Part model, mm, in its own coordinate system. Coordinates: 2 decimals unless noted, no trailing zeros. Loops run counter-clockwise (first coordinate to the right, second up) from the corner with the lowest first, then second, coordinate; pieces in that order, holes last. Notation, with made-up numbers: (39, 71) - (89, 71) arc R18 ccw to (89, 80) - close; hole circle Ø9 at (3, 85). An arc over 180 degrees is marked (long way). Use a Markdown table: item, result. Add a question column.
1) Probe probe 1 along Y at (x, z) = (21, 0.6); probe 2 along Y at (x, z) = (32.5, 2.45); probe 3 along Y at (x, z) = (-3.5, 1.25). List the from-to ranges inside material, lowest first. Write a range as [from, to].
2) Band-saw the part on A-A (x = -6.5). Give the cut face in (y, z) (3 decimals), plus the area to 3 significant figures.
3) Drop flat-ended pins along their axis: P1, Ø1, axis at y = 4, z = 0.5, coming from the +X side; P2, Ø1.6, axis at x = 26, z = 2, coming from the -Y side; P3, Ø6, axis at x = 40.46, y = 60.91, coming from the +Z side. Give the stop position or say it passes through.
4) Band-saw the part on D-D (x = 0). Give the cut face in (y, z) (1 decimal).
5) Band-saw the part on C-C (x = 41). Give the cut face in (y, z) (3 decimals).
6) Band-saw the part on B-B (y = 0). Give the cut face in (x, z) (1 decimal).
from build123d import *

# Parameters (mm, degrees)
SKETCH1_R           = 7.9375
SKETCH1_R_2         = 3.3655
SKETCH1_R_3         = 4.191
BOSS_EXTRUDE1_DEPTH = 3.175
CUT_EXTRUDE1_DEPTH  = 6.35
FILLET1_R           = 3.175
FILLET5_R           = 7.62


with BuildPart() as part:
    # Sketch1 → Boss-Extrude1 (new body)
    with BuildSketch(Plane.XY):
        with BuildLine():
            Line((8.990505701, 142.507164257), (49.453246099, 65.638340515))
            ThreePointArc((49.453246099, 65.638340515), (50.622740399, 60.905856258), (49.453246099, 56.173372001))
            Line((49.453246099, 56.173372001), (8.177790267, -11.326281223))
            ThreePointArc((8.177790267, -11.326281223), (-6.360706327, -12.437938536), (-13.97, 0))
            ThreePointArc((-13.97, 0), (7.91990549, 68.33468047), (-10.16, 137.77468))
            ThreePointArc((-10.16, 137.77468), (-2.437423033, 147.637974022), (8.990505701, 142.507164257))
        make_face()
        Circle(SKETCH1_R, mode=Mode.SUBTRACT)
        with Locations((40.462740399, 60.905856258)):
            Circle(SKETCH1_R_2, mode=Mode.SUBTRACT)
        with Locations((0, 137.77468)):
            Circle(SKETCH1_R_3, mode=Mode.SUBTRACT)
    extrude(amount=BOSS_EXTRUDE1_DEPTH)

    # Sketch2 → Cut-Extrude1 (cut)
    with BuildSketch(Plane.XY.offset(3.175)):
        with BuildLine():
            ThreePointArc((-0.124257687, 11.111805266), (6.119551738, 9.275707131), (10.264347662, 4.258030452))
            Line((10.264347662, 4.258030452), (31.313727824, 38.681050934))
            Line((31.313727824, 38.681050934), (1.961287607, 15.442397513))
            ThreePointArc((1.961287607, 15.442397513), (0.937773258, 13.267826895), (-0.124257687, 11.111805266))
        make_face()
        with BuildLine():
            Line((6.763206822, 27.343322009), (40.914079215, 54.38094756))
            ThreePointArc((40.914079215, 54.38094756), (40.688544415, 54.369255246), (40.462740399, 54.365356258))
            Line((40.462740399, 54.365356258), (13.177274796, 54.365356258))
            ThreePointArc((13.177274796, 54.365356258), (10.666365072, 40.689104041), (6.763206822, 27.343322009))
        make_face()
        with BuildLine():
            Line((14.227692925, 66.924652484), (40.332379532, 67.445056996))
            Line((40.332379532, 67.445056996), (12.691282428, 92.804736539))
            ThreePointArc((12.691282428, 92.804736539), (14.081637817, 79.901629399), (14.227692925, 66.924652484))
        make_face()
        with BuildLine():
            Line((10.611239694, 103.330724773), (36.257061309, 79.801636355))
            Line((36.257061309, 79.801636355), (6.979807085, 135.420906636))
            ThreePointArc((6.979807085, 135.420906636), (4.67858985, 132.085325641), (0.961351613, 130.471683418))
            ThreePointArc((0.961351613, 130.471683418), (6.511625183, 117.159092878), (10.611239694, 103.330724773))
        make_face()
    extrude(amount=-CUT_EXTRUDE1_DEPTH, mode=Mode.SUBTRACT)

    # Fillet1
    # the kernel refuses this fillet: 3.175 mm, written as the material it adds along each edge
    with BuildSketch(Plane(origin=(1.961287607, 15.442397513, 3.175), x_dir=(-0.42030668038784, -0.9073821104812206, 0), z_dir=(0, 0, -1))) as fillet1_piece_1:
        with BuildLine():
            CenterArc((0.755742265, -3.174987871), FILLET1_R, 90.158373023, 26.618624782)
            Line((-0.674656078, -0.340453415), (0, 0))
            ThreePointArc((0, 0), (0.373483081, -0.000516178), (0.746966162, 0))
        make_face()
    extrude(amount=3.175)
    with BuildSketch(Plane(origin=(-0.124257687, 11.111805266, 3.175), x_dir=(0.4359761911813302, 0.8999581994309626, 0), z_dir=(0, 0, -1))) as fillet1_piece_2:
        with BuildLine():
            CenterArc((4.22998716, 3.174619998), FILLET1_R, 172.83641486, 96.277116616)
            ThreePointArc((1.07977071, 3.570550945), (0.690776023, 1.739644609), (0, 0))
            ThreePointArc((0, 0), (2.090433086, 0.016171698), (4.180866173, 0))
        make_face()
    extrude(amount=3.175)
    with BuildSketch(Plane(origin=(10.264347662, 4.258030452, 3.175), x_dir=(0.5216861951219568, 0.853137453063207, 0), z_dir=(0, 0, -1))) as fillet1_piece_3:
        with BuildLine():
            CenterArc((4.899209013, -3.175), FILLET1_R, 90, 103.603922827)
            ThreePointArc((1.813283958, -3.921787493), (1.099083544, -1.871916155), (0, 0))
            Line((0, 0), (4.899209013, 0))
        make_face()
    extrude(amount=3.175)
    with BuildSketch(Plane(origin=(31.313727824, 38.681050934, 3.175), x_dir=(-0.7840288614357019, -0.6207243707442435, 0), z_dir=(0, 0, -1))) as fillet1_piece_4:
        with BuildLine():
            CenterArc((FILLET1_R * 5.61807899766, -FILLET1_R), FILLET1_R, 90, 159.814477423)
            Line((FILLET1_R * 5.27301794688, -FILLET1_R * 1.9385802423), (0, 0))
            Line((0, 0), (FILLET1_R * 5.61807899766, 0))
        make_face()
    extrude(amount=3.175)
    with BuildSketch(Plane(origin=(40.914079215, 54.38094756, 3.175), x_dir=(-0.9999985466583668, -0.0017048991624346568, 0), z_dir=(0, 0, -1))) as fillet1_piece_5:
        with BuildLine():
            CenterArc((9.150412322, -3.174995386), FILLET1_R, 90.097683574, 141.630948821)
            Line((7.1838593, -5.667643418), (6.987203998, -5.916908221))
            Line((6.987203998, -5.916908221), (-0.196655302, -0.249264803))
            Line((-0.196655302, -0.249264803), (0.021369604, 0.316780034))
            ThreePointArc((0.021369604, 0.316780034), (0.450823437, 0.302677747), (9.144457961, 0.317499539))
            Line((9.144457961, 0.317499539), (9.144999267, 0))
        make_face()
    extrude(amount=3.175)
    with BuildSketch(Plane(origin=(6.763206822, 27.343322009, 3.175), x_dir=(0.29421486221715376, 0.9557393027654252, 0), z_dir=(0, 0, -1))) as fillet1_piece_6:
        with BuildLine():
            CenterArc((10.215496918, 3.172783065), FILLET1_R, 124.520485767, 143.338263429)
            Line((8.41622168, 5.788740561), (0, 0))
            ThreePointArc((0, 0), (5.048434414, 0.094345715), (10.096868828, 0))
        make_face()
    extrude(amount=3.175)
    with BuildSketch(Plane(origin=(13.177274796, 54.365356258, 3.175), x_dir=(-0.1397274976091422, -0.9901899951079526, 0), z_dir=(0, 0, -1))) as fillet1_piece_7:
        with BuildLine():
            CenterArc((2.758448164, -3.174838407), FILLET1_R, 90.57806828, 81.3898537)
            Line((-0.38540507, -2.731203602), (0, 0))
            ThreePointArc((0, 0), (1.363207757, -0.006876893), (2.726415514, 0))
        make_face()
    extrude(amount=3.175)
    with BuildSketch(Plane(origin=(12.691282428, 92.804736539, 3.175), x_dir=(0.12348134501551586, -0.992346893698549, 0), z_dir=(0, 0, -1))) as fillet1_piece_8:
        with BuildLine():
            CenterArc((8.634113181, -3.173416471), FILLET1_R, 91.809659599, 137.818629886)
            Line((6.577526563, -5.59231632), (0, 0))
            ThreePointArc((0, 0), (4.266924504, -0.06738998), (8.533849008, 0))
        make_face()
    extrude(amount=3.175)
    with BuildSketch(Plane(origin=(14.227692925, 66.924652484, 3.175), x_dir=(0.024643115282951916, 0.9996963123214726, 0), z_dir=(0, 0, -1))) as fillet1_piece_9:
        with BuildLine():
            CenterArc((3.319776694, 3.174765946), FILLET1_R, 177.445853815, 91.858439002)
            Line((0.147930885, 3.316255051), (0, 0))
            ThreePointArc((0, 0), (1.640612791, 0.009960595), (3.281225581, 0))
        make_face()
    extrude(amount=3.175)
    with BuildSketch(Plane(origin=(40.332379532, 67.445056996, 3.175), x_dir=(-0.7368618420904852, 0.6760433607920552, 0), z_dir=(0, 0, -1))) as fillet1_piece_10:
        with BuildLine():
            CenterArc((FILLET1_R * 2.49529647453, -FILLET1_R), FILLET1_R, 90, 136.322717601)
            Line((FILLET1_R * 1.80470077201, -FILLET1_R * 1.72324102183), (0, 0))
            Line((0, 0), (FILLET1_R * 2.49529647453, 0))
        make_face()
    extrude(amount=3.175)
    with BuildSketch(Plane(origin=(36.257061309, 79.801636355, 3.175), x_dir=(-0.736861842090485, 0.6760433607920552, 0), z_dir=(0, 0, -1))) as fillet1_piece_11:
        with BuildLine():
            CenterArc((FILLET1_R * 5.75850458875, FILLET1_R), FILLET1_R, 109.70304414, 160.29695586)
            Line((FILLET1_R * 5.42135931021, FILLET1_R * 1.94145263352), (0, 0))
            Line((0, 0), (FILLET1_R * 5.75850458875, 0))
        make_face()
    extrude(amount=3.175)
    with BuildSketch(Plane(origin=(10.611239694, 103.330724773, 3.175), x_dir=(0.7368618420904525, -0.6760433607920909, 0), z_dir=(0, 0, -1))) as fillet1_piece_12:
        with BuildLine():
            CenterArc((0.964871334, -3.175), FILLET1_R, 90, 33.606646982)
            ThreePointArc((-0.792453619, -0.530678913), (-0.395758583, -0.266038651), (0, 0))
            Line((0, 0), (0.964871334, 0))
        make_face()
    extrude(amount=3.175)
    with BuildSketch(Plane(origin=(0.961351613, 130.471683418, 3.175), x_dir=(0.42205519537851754, -0.9065701363126856, 0), z_dir=(0, 0, -1))) as fillet1_piece_13:
        with BuildLine():
            CenterArc((3.47040448, -3.174744224), FILLET1_R, 90.727275071, 84.025505032)
            ThreePointArc((0.308709742, -2.884379996), (0.297748154, -1.426842886), (0, 0))
            ThreePointArc((0, 0), (1.715052097, -0.01088502), (3.430104193, 0))
        make_face()
    extrude(amount=3.175)
    with BuildSketch(Plane(origin=(6.979807085, 135.420906636, 3.175), x_dir=(-0.5768732919878915, -0.8168336458490512, 0), z_dir=(0, 0, -1))) as fillet1_piece_14:
        with BuildLine():
            CenterArc((5.114466288, -3.042745801), FILLET1_R, 106.595474978, 100.411869016)
            Line((2.285705354, -4.484528231), (0, 0))
            ThreePointArc((0, 0), (2.103823012, -0.306829742), (4.207646024, 0))
        make_face()
    extrude(amount=3.175)

    # Fillet5
    # the kernel refuses this fillet: 7.62 mm, written as the material it takes off along each edge
    with BuildSketch(Plane(origin=(49.453246099, 56.173372001, -1.634441158), x_dir=(0.4370839848417488, 0.8994206970016078, 0), z_dir=(0, 0, 1))) as fillet5_piece_1:
        with BuildLine():
            CenterArc((0.40861029, 7.616054986), FILLET5_R, 264.472549142, 7.371205669)
            Line((-0.325368255, 0.031486739), (0, 0))
            ThreePointArc((0, 0), (0.326888232, -0.005260019), (0.653776463, 0))
        make_face()
    extrude(amount=6.443882317, mode=Mode.SUBTRACT)
    with BuildSketch(Plane(origin=(8.177790267, -11.326281223, -6.850611907), x_dir=(-0.8642606797046686, -0.5030442103000734, 0), z_dir=(0, 0, 1))) as fillet5_piece_2:
        with BuildLine():
            CenterArc((1.992905282, -7.583263394), FILLET5_R, 84.371608536, 33.981356684)
            Line((-1.625847463, -0.877368333), (0, 0))
            ThreePointArc((0, 0), (1.370122381, 0.067350445), (2.740244763, 0))
        make_face()
    extrude(amount=16.876223814, mode=Mode.SUBTRACT)
    with BuildSketch(Plane(origin=(-13.97, 0, -10.334031649), x_dir=(0.5495701737634485, 0.8354475591619218, 0), z_dir=(0, 0, 1))) as fillet5_piece_3:
        with BuildLine():
            CenterArc((2.78803259, -7.619578759), FILLET5_R, 90.602458764, 49.750903142)
            ThreePointArc((-3.079322695, -2.757630389), (-1.64222079, -1.264291645), (0, 0))
            ThreePointArc((0, 0), (1.353955306, -0.00711841), (2.707910612, 0))
        make_face()
    extrude(amount=23.843063299, mode=Mode.SUBTRACT)
    with BuildSketch(Plane(origin=(-10.16, 137.77468, -14.229821855), x_dir=(0.28011460344612044, 0.9599665665720981, 0), z_dir=(0, 0, 1))) as fillet5_piece_4:
        with BuildLine():
            CenterArc((3.557455464, -7.314945237), FILLET5_R, 73.732955283, 62.075524842)
            ThreePointArc((-1.906189574, -2.003355748), (-0.947716818, -1.006795003), (0, 0))
            ThreePointArc((0, 0), (2.845964371, 0.406739684), (5.691928742, 0))
        make_face()
    extrude(amount=31.63464371, mode=Mode.SUBTRACT)


solid = part.part
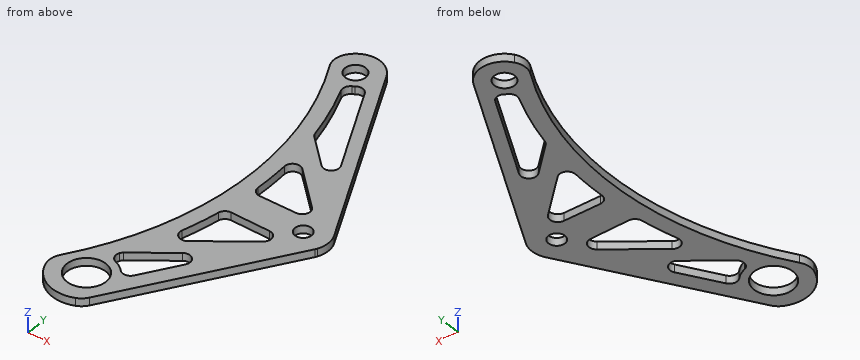
Answer block:
| question | item | result |
|---|---|---|
| 1 | probe 1 | [9.64, 21.81], [27.8, 38.61], [54.37, 67.06], [85.18, 93.8], [108.79, 119.69] |
| 1 | probe 2 | [28.45, 47.72], [54.28, 67.29], [74.63, 97.85] |
| 1 | probe 3 | [-13.52, -7.12], [7.12, 18.77], [125.02, 135.47], [140.08, 147.31] |
| 2 | outline | (-12.366, 0) - (-4.556, 0) - (-4.556, 3.175) - (-12.366, 3.175) - close; (4.556, 0) - (12.59, 0) - (12.59, 3.175) - (4.556, 3.175) - close; (131.198, 0) - (145.583, 0) - (145.583, 3.175) - (131.198, 3.175) - close |
| 2 | area | 96.0 mm2 |
| 3 | P1 | x = 17.86 |
| 3 | P2 | y = 16.51 |
| 3 | P3 | through |
| 4 | outline | (-14, 0) - (-7.9, 0) - (-7.9, 3.2) - (-14, 3.2) - close; (7.9, 0) - (27.3, 0) - (27.3, 3.2) - (7.9, 3.2) - close; (116.5, 0) - (133.6, 0) - (133.6, 3.2) - (116.5, 3.2) - close; (142, 0) - (147.9, 0) - (147.9, 3.2) - (142, 3.2) - close |
| 5 | outline | (42.349, 0) - (57.584, 0) - (57.584, 3.175) - (42.349, 3.175) - close; (64.228, 0) - (81.697, 0) - (81.697, 3.175) - (64.228, 3.175) - close |
| 6 | outline | (-13.5, 0) - (-7.9, 0) - (-7.9, 3.2) - (-13.5, 3.2) - close; (7.9, 0) - (15.1, 0) - (15.1, 3.2) - (7.9, 3.2) - close |
